The listing builds one solid part. Answer for the finished solid, in the listing's coordinates (mm). Face numbers are marked on the shaded views. A direction names the side the tool comes from. Round coordinates to 2 decimals unless told otherwise and drop trailing zeros. Write each loop counter-clockwise with the first axis right and the second up, starting at its lowest first coordinate (ties: lowest second). Pieces come first, ordered by that corner, then holes. Notation, with made-up numbers: M 2,52 L 54,52 A18 cw 54,59 Z; hole C 79,-26.5 d8. An arc over 180 degrees is marked long. Write each question's results on one line, items separated by ' | '.
from build123d import *

# Parameters (mm, degrees)
F1_W          = 38.4
F1_H          = 38.4
F1_W_2        = 36.4
F1_H_2        = 36.4
F2_DEPTH      = 11.8
F3_R          = 1.5
F3_W          = 38.4
F3_H          = 38.4
F3_W_2        = 36.4
F3_H_2        = 36.4
F4_DEPTH      = 2
F4_DEPTH_BACK = 1
F5_R          = 0.6
F6_W          = 8
F6_H          = 1
F7_DEPTH      = 0.5


with BuildPart() as f2:
    # F1 (on Top) → F2 (new body)
    with BuildSketch(Plane.XY):
        Rectangle(F1_W, F1_H)
        Rectangle(F1_W_2, F1_H_2, mode=Mode.SUBTRACT)
    extrude(amount=F2_DEPTH)

    # F3 (on face) → F4 (join, two sides)
    with BuildSketch(Plane.XY.offset(11.8)) as f4_sk:
        with BuildLine():
            ThreePointArc((-35, -46.5), (-34.12132, -48.62132), (-32, -49.5))
            Line((-32, -49.5), (-22, -49.5))
            ThreePointArc((-22, -49.5), (-19.87868, -48.62132), (-19, -46.5))
            Line((-19, -46.5), (-19, -45.438493))
            ThreePointArc((-19, -45.438493), (-18.950318, -44.894781), (-18.802918, -44.369078))
            Line((-18.802918, -44.369078), (-13.230511, -29.763898))
            ThreePointArc((-13.230511, -29.763898), (-12.151972, -28.06913), (-10.493455, -26.935637))
            Line((-10.493455, -26.935637), (-3.057386, -23.81569))
            ThreePointArc((-3.057386, -23.81569), (0.049323, -23.192689), (3.154219, -23.824657))
            Line((3.154219, -23.824657), (10.503716, -26.933267))
            ThreePointArc((10.503716, -26.933267), (12.153945, -28.066345), (13.227468, -29.755923))
            Line((13.227468, -29.755923), (18.802918, -44.369078))
            ThreePointArc((18.802918, -44.369078), (18.950318, -44.894781), (19, -45.438493))
            Line((19, -45.438493), (19, -46.5))
            ThreePointArc((19, -46.5), (19.87868, -48.62132), (22, -49.5))
            Line((22, -49.5), (32, -49.5))
            ThreePointArc((32, -49.5), (34.12132, -48.62132), (35, -46.5))
            Line((35, -46.5), (35, -44.801084))
            ThreePointArc((35, -44.801084), (34.484786, -43.120061), (33.116107, -42.016429))
            ThreePointArc((33.116107, -42.016429), (31.618403, -41.017341), (30.649398, -39.5))
            Line((30.649398, -39.5), (26.524716, -28.620354))
            ThreePointArc((26.524716, -28.620354), (26.281849, -27.748859), (26.2, -26.847865))
            Line((26.2, -26.847865), (26.2, 11.797695))
            ThreePointArc((26.2, 11.797695), (27.038254, 14.568952), (29.271947, 16.411003))
            Line((29.271947, 16.411003), (33.054434, 17.991828))
            ThreePointArc((33.054434, 17.991828), (34.344715, 19.024405), (34.892422, 20.58359))
            Line((34.892422, 20.58359), (34.99482, 22.323777))
            ThreePointArc((34.99482, 22.323777), (34.18231, 24.558524), (31.99876, 25.5))
            Line((31.99876, 25.5), (21.997216, 25.495866))
            ThreePointArc((21.997216, 25.495866), (20.678268, 25.189768), (19.628246, 24.334917))
            ThreePointArc((19.628246, 24.334917), (17.87728, 22.90971), (15.677896, 22.4))
            Line((15.677896, 22.4), (-15.677896, 22.4))
            ThreePointArc((-15.677896, 22.4), (-17.87728, 22.90971), (-19.628246, 24.334917))
            ThreePointArc((-19.628246, 24.334917), (-20.678268, 25.189768), (-21.997216, 25.495866))
            Line((-21.997216, 25.495866), (-31.99876, 25.5))
            ThreePointArc((-31.99876, 25.5), (-34.18231, 24.558524), (-34.99482, 22.323777))
            Line((-34.99482, 22.323777), (-34.892422, 20.58359))
            ThreePointArc((-34.892422, 20.58359), (-34.344715, 19.024405), (-33.054434, 17.991828))
            Line((-33.054434, 17.991828), (-29.271947, 16.411003))
            ThreePointArc((-29.271947, 16.411003), (-27.038254, 14.568952), (-26.2, 11.797695))
            Line((-26.2, 11.797695), (-26.2, -26.847865))
            ThreePointArc((-26.2, -26.847865), (-26.281849, -27.748859), (-26.524716, -28.620354))
            Line((-26.524716, -28.620354), (-30.649398, -39.5))
            ThreePointArc((-30.649398, -39.5), (-31.618403, -41.017341), (-33.116107, -42.016429))
            ThreePointArc((-33.116107, -42.016429), (-34.484786, -43.120061), (-35, -44.801084))
            Line((-35, -44.801084), (-35, -46.5))
        make_face()
        with Locations((-32, -46.5)):
            Circle(F3_R, mode=Mode.SUBTRACT)
        with Locations((-22, -46.5)):
            Circle(F3_R, mode=Mode.SUBTRACT)
        with Locations((22, -46.5)):
            Circle(F3_R, mode=Mode.SUBTRACT)
        with Locations((32, -46.5)):
            Circle(F3_R, mode=Mode.SUBTRACT)
        with BuildLine():
            ThreePointArc((-20.5, -17.5), (-22, -19), (-23.5, -17.5))
            Line((-23.5, -17.5), (-23.5, 17.5))
            ThreePointArc((-23.5, 17.5), (-22, 19), (-20.5, 17.5))
            Line((-20.5, 17.5), (-20.5, -17.5))
        make_face(mode=Mode.SUBTRACT)
        with Locations((-32, 22.5)):
            Circle(F3_R, mode=Mode.SUBTRACT)
        with Locations((-21.998456, 22.495866)):
            Circle(F3_R, mode=Mode.SUBTRACT)
        Rectangle(F3_W, F3_H, mode=Mode.SUBTRACT)
        with BuildLine():
            ThreePointArc((20.5, 17.5), (22, 19), (23.5, 17.5))
            Line((23.5, 17.5), (23.5, -17.5))
            ThreePointArc((23.5, -17.5), (22, -19), (20.5, -17.5))
            Line((20.5, -17.5), (20.5, 17.5))
        make_face(mode=Mode.SUBTRACT)
        with Locations((22, 22.5)):
            Circle(F3_R, mode=Mode.SUBTRACT)
        with Locations((32, 22.5)):
            Circle(F3_R, mode=Mode.SUBTRACT)
        Rectangle(F3_W, F3_H)
        Rectangle(F3_W_2, F3_H_2, mode=Mode.SUBTRACT)
    extrude(amount=F4_DEPTH)
    extrude(f4_sk.sketch, amount=-F4_DEPTH_BACK)

    # F5
    f5_edges = [f2.edges().sort_by_distance(p)[0] for p in [
        (-19.2, -19.2, 5.4),
        (19.2, -19.2, 5.4),
        (19.2, 19.2, 5.4),
        (-19.2, 19.2, 5.4),
    ]]
    fillet(f5_edges, radius=F5_R)

    # F6 (on face) → F7 (cut)
    with BuildSketch(Plane.XY.offset(13.8)):
        with Locations((-22.2, 0)):
            Rectangle(F6_W, F6_H)
        with Locations((22.2, 0)):
            Rectangle(F6_W, F6_H)
    extrude(amount=-F7_DEPTH, mode=Mode.SUBTRACT)


solid = f2.part
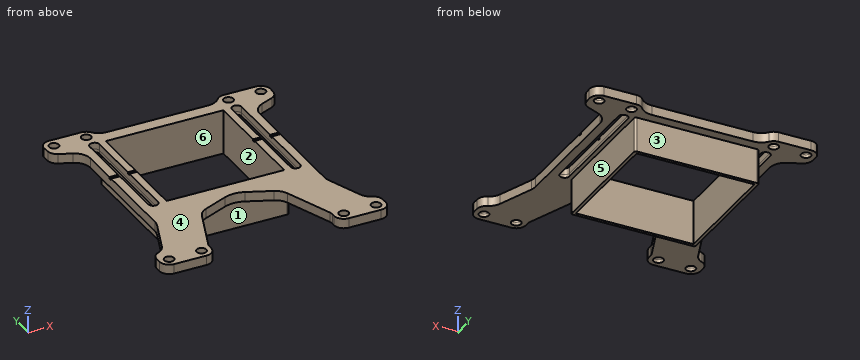
1) Section D-D (x = -6) is taken. Determine the outline of the cut face in (y, z), then the cut area to 3 significant figures.
Return value:
outline: M -25.05,10.8 L -19.2,10.8 L -19.2,0 L -18.2,0 L -18.2,13.8 L -25.05,13.8 Z; M 18.2,0 L 19.2,0 L 19.2,10.8 L 22.4,10.8 L 22.4,13.8 L 18.2,13.8 Z | area: 54.8 mm²
2) Section B-B (x = 14.5) is taken. Determine the outline of the cut face in (y, z).
Return value:
outline: M -33.09,10.8 L -19.2,10.8 L -19.2,0 L -18.2,0 L -18.2,13.8 L -33.09,13.8 Z; M 18.2,0 L 19.2,0 L 19.2,10.8 L 22.4,10.8 L 22.4,13.8 L 18.2,13.8 Z
3) Section C-C (z = 4) is taken. Determine the outline of the cut face in (x, y).
Return value:
outline: M -19.2,-18.6 A0.6 ccw -18.6,-19.2 L 18.6,-19.2 A0.6 ccw 19.2,-18.6 L 19.2,18.6 A0.6 ccw 18.6,19.2 L -18.6,19.2 A0.6 ccw -19.2,18.6 Z; hole M -18.2,-18.2 L 18.2,-18.2 L 18.2,18.2 L -18.2,18.2 Z
4) The mould has two halves that part along X. Classify the marked faces 4, 5 and 6: +X half, -X half, draft (parallel to the pull), parting line (faces both ways), or undercut.
Return value:
face 4: draft | face 5: +X half | face 6: undercut
5) Section A-A (y = -13) is taken. Determine the outline of the cut face in (x, z), then the cut area to 3 significant figures.
Return value:
outline: M -26.2,10.8 L -23.5,10.8 L -23.5,13.8 L -26.2,13.8 Z; M -20.5,10.8 L -19.2,10.8 L -19.2,0 L -18.2,0 L -18.2,13.8 L -20.5,13.8 Z; M 18.2,0 L 19.2,0 L 19.2,10.8 L 20.5,10.8 L 20.5,13.8 L 18.2,13.8 Z; M 23.5,10.8 L 26.2,10.8 L 26.2,13.8 L 23.5,13.8 Z | area: 51.6 mm²
6) Find the intervals of material crossed by line 1 (Y direction, x = 22, z = 12.55); line 2 (X direction, y = -15.5, z = 6.75), in increasing order.
Return value:
line 1: -49.5 to -48, -45 to -19, 19 to 21, 24 to 25.5 | line 2: -19.2 to -18.2, 18.2 to 19.2
7) Each of these flat-tipped pins is pushed along its axis until it touches: pin 1 (4 mm diameter, centred on x = 22, y = 22.5, fed in from -Z); pin 2 (0.5 mm diameter, centred on y = -1.5, z = 11, fed in from +X); pin 3 (2.5 mm diameter, centred on x = -32, y = -46.5, fed in from -Z); pin 4 (0.6 mm diameter, centred on y = -6, z = 12.5, fed in from -X). Where does it stop, or does it pass through?
Return value:
pin 1: z = 10.8 | pin 2: x = 26.2 | pin 3: through | pin 4: x = -26.2
8) A tool of negligible diameter and unlimited length cuts with its end or side. For the marked faces 1, 2 and 3, from which of +Z, -Z, +X, -X, +Y, -Y can it reach the whole face along a straight path? Write none if from no direction.
Return value:
face 1: -Z, +X, -X, -Y | face 2: +Z, -Z | face 3: -Z, +X, -X, +Y
